from build123d import *

# Parameters (mm, degrees)
F0_R     = 2.5
F0_R_2   = 2
F1_DEPTH = 6
F2_DEPTH = 3.2
F3_R     = 9.99999


# Not quite as in the source:
# - a fillet or chamfer is up to 0.001 mm smaller than in the source, because OpenCascade refuses the exact size


with BuildPart() as f1:
    # F0 (on Top) → F1 (new body)
    with BuildSketch(Plane.XY):
        Polygon((20, -10), (20, 10), (0, 10), (-20, 10), (-20, -10), (0, -10), align=None)
        Polygon((-10, 4.0414518843), (-6.5, 2.0207259422), (-6.5, -2.0207259422), (-10, -4.0414518843), (-13.5, -2.0207259422), (-13.5, 2.0207259422), align=None, mode=Mode.SUBTRACT)
        with Locations((10, 0)):
            Circle(F0_R, mode=Mode.SUBTRACT)
        Polygon((-6.5, -2.0207259422), (-6.5, 2.0207259422), (-10, 4.0414518843), (-13.5, 2.0207259422), (-13.5, -2.0207259422), (-10, -4.0414518843), align=None)
        with Locations((-10, 0)):
            Circle(F0_R_2, mode=Mode.SUBTRACT)
    extrude(amount=F1_DEPTH)

    # F0 (on Top) → F2 (cut)
    with BuildSketch(Plane.XY):
        Polygon((-6.5, -2.0207259422), (-6.5, 2.0207259422), (-10, 4.0414518843), (-13.5, 2.0207259422), (-13.5, -2.0207259422), (-10, -4.0414518843), align=None)
        with Locations((-10, 0)):
            Circle(F0_R_2, mode=Mode.SUBTRACT)
    extrude(amount=F2_DEPTH, mode=Mode.SUBTRACT)

    # F3 (radius 10 in the source; OpenCascade refuses exactly that, so slightly less here)
    f3_edges = [f1.edges().sort_by_distance(p)[0] for p in [
        (-20, -10, 3),
        (20, -10, 3),
        (20, 10, 3),
        (-20, 10, 3),
    ]]
    fillet(f3_edges, radius=F3_R)


solid = f1.part
Build history of the part. All positions in model axes, mm. A direction names the side the tool comes from. Round coordinates to 2 decimals unless told otherwise and drop trailing zeros. Write each loop counter-clockwise with the first axis right and the second up, starting at its lowest first coordinate (ties: lowest second). Pieces come first, ordered by that corner, then holes. Notation, with made-up numbers: (46, -9) - (59, -9) arc R22 ccw to (59, 13) - close; hole circle Ø3 at (46, -23.75). An arc over 180 degrees is marked (long way). Use CSV: the item, a comma, the result in double quotes.
(1) Band-saw the part on A-A (z = 4.5). Give the number of separate pieces and of enclosed holes in the cut face, plus the area to 3 significant figures.
Response:
separate pieces,"1"
enclosed holes,"2"
area,"682 mm²"
(2) Pin check, flat tips, straight feed: P1, Ø8, axis at x = -0.5, y = -2, coming from the -Z side; P2, Ø3, axis at x = 12, z = 3, coming from the -Y side. Stop position of each tip, or through.
Response:
P1,"z = 0"
P2,"y = -9.99"
(3) Band-saw the part on B-B (x = 12). Write the cut outline in (y, z).
Response:
outline,"(-9.8, 0) - (-1.5, 0) - (-1.5, 6) - (-9.8, 6) - close; (1.5, 0) - (9.8, 0) - (9.8, 6) - (1.5, 6) - close"
(4) 3-axis set-ups, long thin cutter, end or side, ignore diameter. For faces 1 (the flat face through (-11.8, -3, 1.6)), 2 (the flat face through (0, 10, 3)): which of +Z, -Z, +X, -X, +Y, -Y reach the whole face in a straight line?
Response:
face 1,"-Z"
face 2,"+Z, -Z, +X, -X, +Y"
(5) Wall check: line 1 (Y direction, x = -10, z = 5.45); line 2 (Y direction, x = 10, z = 1.7); line 3 (X direction, y = -0.75, z = 5.05). Give the ranges that are in metal, low to high.
Response:
line 1,"-10 to -2, 2 to 10"
line 2,"-10 to -2.5, 2.5 to 10"
line 3,"-19.97 to -11.85, -8.15 to 7.62, 12.38 to 19.97"
(6) Mould opens along X. For faces 3 (the cylindrical face through (-16.99, -7.15, 3.04)), 4 (the flat face through (-6.5, 0, 2)), 5 (the flat face through (0, -10, 3)) say: pulls with the +X half, pulls with the -X half, needs draft (parallel to the pull), parting line crosses it, or undercut.
Response:
face 3,"pulls with the -X half"
face 4,"undercut"
face 5,"needs draft"
(7) Band-saw the part on D-D (y = -8). Write the cut outline in (x, z), plus the area to 3 significant figures.
Response:
outline,"(-16, 0) - (16, 0) - (16, 6) - (-16, 6) - close"
area,"192 mm²"
